The model under review builds one solid part; all positions refer to its coordinate system, in mm. A direction names the side the tool comes from. Coordinates: 2 decimals unless noted, no trailing zeros. Order: outer loops, then holes, each group sorted by start corner. A loop starts at its lowest first (then second) coordinate and runs counter-clockwise, first axis right, second up. Notation, with made-up numbers: M 49,6 L 59,6 A29 ccw 59,28 Z; hole C 77,-7.75 d10. An arc over 180 degrees is marked long. One line per item, written item: value.
```python
from build123d import *

# Parameters (mm, degrees)
CROQUIS1_R                 = 1.5
SALIENTE_EXTRUIR1_DEPTH    = 7
CORTAR_EXTRUIR1_DEPTH      = 13
CORTAR_EXTRUIR1_DEPTH_BACK = 27.438608133
CROQUIS2_R                 = 1.5
CORTAR_EXTRUIR2_DEPTH      = 27.438608133
CORTAR_EXTRUIR2_DEPTH_BACK = 27.438608133
CROQUIS3_W                 = 5
CROQUIS3_H                 = 7
CORTAR_EXTRUIR3_DEPTH      = 1.5
CROQUIS5_W                 = 3
CROQUIS5_H                 = 6
CORTAR_EXTRUIR4_DEPTH      = 27.438608133


with BuildPart() as part:
    # Croquis1 → Saliente-Extruir1 (new, symmetric)
    with BuildSketch(Plane(origin=(0, 0, 0), x_dir=(0, 0, -1), z_dir=(1, 0, 0))):
        with BuildLine():
            Line((-24, 5), (15, 5))
            Line((15, 5), (15, -5))
            Line((15, -5), (-24, -5))
            ThreePointArc((-24, -5), (-24.707106781, -4.707106781), (-25, -4))
            Line((-25, -4), (-25, 4))
            ThreePointArc((-25, 4), (-24.707106781, 4.707106781), (-24, 5))
        make_face()
        with Locations((-22, 0)):
            Circle(CROQUIS1_R, mode=Mode.SUBTRACT)
    extrude(amount=SALIENTE_EXTRUIR1_DEPTH, both=True)

    # Croquis2 → Cortar-Extruir1 (cut, two sides: drawn at the far end of the back side and taken through both)
    with BuildSketch(Plane.XY.offset(-CORTAR_EXTRUIR1_DEPTH_BACK)):
        with Locations(Location((0, 0, 0), (0, 0, 180))):
            Circle(CROQUIS2_R)
    extrude(amount=CORTAR_EXTRUIR1_DEPTH + CORTAR_EXTRUIR1_DEPTH_BACK, mode=Mode.SUBTRACT)

    # Croquis3 → Cortar-Extruir2 (cut, two sides: drawn at the far end of the back side and taken through both)
    with BuildSketch(Plane(origin=(0, 0, 0), x_dir=(1, 0, 0), z_dir=(0, 1, 0)).offset(-CORTAR_EXTRUIR2_DEPTH_BACK)):
        with Locations((0, -21.5)):
            Rectangle(CROQUIS3_W, CROQUIS3_H)
    extrude(amount=CORTAR_EXTRUIR2_DEPTH + CORTAR_EXTRUIR2_DEPTH_BACK, mode=Mode.SUBTRACT)

    # Croquis4 → Cortar-Extruir3 (cut, symmetric)
    with BuildSketch(Plane.XY):
        Polygon((1.732050808, 3), (-1.732050808, 3), (-3.464101615, 0), (-1.732050808, -3), (1.732050808, -3), (3.464101615, 0), align=None)
    extrude(amount=CORTAR_EXTRUIR3_DEPTH, both=True, mode=Mode.SUBTRACT)

    # Croquis5 → Cortar-Extruir4 (cut, through all)
    with BuildSketch(Plane(origin=(0, 0, 0), x_dir=(0, 0, -1), z_dir=(1, 0, 0))):
        Rectangle(CROQUIS5_W, CROQUIS5_H)
    extrude(amount=-CORTAR_EXTRUIR4_DEPTH, mode=Mode.SUBTRACT)


solid = part.part
```
(1) We need section C-C, the plane y = 3.5. State the section outline as (x, z) points, plus the area to 3 significant figures.
Geometry results:
outline: M -7,-15 L 7,-15 L 7,25 L 2.5,25 L 2.5,18 L -2.5,18 L -2.5,25 L -7,25 Z
area: 525 mm2
(2) Insertion check: pin 1 Ø0.9 at (x, y) = (-0.5, 0) entering from -Z; pin 2 Ø2.5 at (y, z) = (0, 22) entering from +X (3 decimals); pin 3 Ø1.8 at (x, y) = (0, 0) entering from +Z; pin 4 Ø4 at (x, y) = (-1, -0.5) entering from +Z. Each pin has a flat end and moves straight along its axis. Give the tip position at first contact, or say it passes through.
Geometry results:
pin 1: stops at z = 13
pin 2: passes through
pin 3: stops at z = 18
pin 4: stops at z = 25
(3) Tool access review of faces 1 (the flat face through (0, 0, 13)), 2 (the flat face through (-3, 0, -1.5)), 3 (the flat face through (0, 0, 18)): name each direction out of +Z, -Z, +X, -X, +Y, -Y from which nothing blocks a thin tool from reaching the whole face with its end or side.
Geometry results:
face 1: -Z
face 2: -X
face 3: +Z, +Y, -Y
(4) Mouldability with a two-part tool opening along X and no side actions: class faces 4 (the flat face through (-7, 0, 5)), 5 (the flat face through (-3, 3, 0)), 6 (the flat face through (7, 0, 5)), 7 (the flat face through (2.5, -1.2, 20.8)) as +X half, -X half, draft (parallel to the pull), parting line (faces both ways), or undercut.
Geometry results:
face 4: -X half
face 5: draft
face 6: +X half
face 7: undercut
(5) We need section D-D, the plane y = 0.75. State the section outline as (x, z) points, plus the area to 3 significant figures.
Geometry results:
outline: M -7,-15 L -1.3,-15 L -1.3,-1.5 L -7,-1.5 Z; M -7,1.5 L -1.3,1.5 L -1.3,13 L 1.3,13 L 1.3,1.5 L 3.03,1.5 L 3.03,-1.5 L 1.3,-1.5 L 1.3,-15 L 7,-15 L 7,20.7 L 2.5,20.7 L 2.5,18 L -2.5,18 L -2.5,20.7 L -7,20.7 Z; M -7,23.3 L -2.5,23.3 L -2.5,25 L -7,25 Z; M 2.5,23.3 L 7,23.3 L 7,25 L 2.5,25 Z
area: 407 mm2
(6) We need section B-B, the plane x = 5.75. State the section outline as (y, z) points.
Geometry results:
outline: M -5,-15 L 5,-15 L 5,24 A1 ccw 4,25 L -4,25 A1 ccw -5,24 Z; hole C 0,22 d3
(7) We need section A-A, the plane z = 22. State the section outline as (x, y) points, plus the area to 3 significant figures.
Geometry results:
outline: M -7,-5 L -2.5,-5 L -2.5,-1.5 L -7,-1.5 Z; M -7,1.5 L -2.5,1.5 L -2.5,5 L -7,5 Z; M 2.5,-5 L 7,-5 L 7,-1.5 L 2.5,-1.5 Z; M 2.5,1.5 L 7,1.5 L 7,5 L 2.5,5 Z
area: 63.0 mm2
(8) For L1, parallel to Z at x = -5.45, y = 0; L2, parallel to Y at x = 0, z = 10.25; L3, parallel to Z at x = 1, y = 1.5, list the stretches that pass through material, from the lowest coordinate up.
Geometry results:
L1: z = -15 to -1.5, 1.5 to 20.5, 23.5 to 25
L2: y = -5 to -1.5, 1.5 to 5
L3: z = -15 to -1.5, 1.5 to 18
